Can you work these out from the model? Positions are in its coordinate system, mm. A direction names the side the tool comes from. Round coordinates to 2 decimals unless told otherwise and drop trailing zeros. Loops run counter-clockwise (first coordinate to the right, second up) from the corner with the lowest first, then second, coordinate; pieces in that order, holes last. Notation, with made-up numbers: (34.5, 2) -> (60.5, 2) arc R20 cw to (60.5, 14) -> close; hole circle Ø5 at (-29.5, 74). An arc over 180 degrees is marked (long way). Answer as a JSON object with one key per item and string values.
```python
from build123d import *

# Parameters (mm, degrees)
SKETCH_1_W          = 40
SKETCH_1_H          = 24
SKETCH_1_R          = 2
EXTRUDE_1_DEPTH     = 3
SKETCH_2_W          = 20
SKETCH_2_H          = 6
EXTRUDE_2_DEPTH     = 25
SKETCH_3_R          = 7.9375
CUT_EXTRUDE_1_DEPTH = 10


with BuildPart() as part:
    # 草图1 → 凸台-拉伸1 (new body)
    with BuildSketch(Plane(origin=(0, 0, 0), x_dir=(1, 0, 0), z_dir=(0, 1, 0))):
        Rectangle(SKETCH_1_W, SKETCH_1_H)
        with Locations((-14.8, -7.5)):
            Circle(SKETCH_1_R, mode=Mode.SUBTRACT)
        with Locations((14.8, -7.5)):
            Circle(SKETCH_1_R, mode=Mode.SUBTRACT)
        with Locations((-14.8, 7.5)):
            Circle(SKETCH_1_R, mode=Mode.SUBTRACT)
        with Locations((14.8, 7.5)):
            Circle(SKETCH_1_R, mode=Mode.SUBTRACT)
    extrude(amount=EXTRUDE_1_DEPTH)

    # 草图2 → 凸台-拉伸2 (add)
    with BuildSketch(Plane(origin=(0, 3, 0), x_dir=(1, 0, 0), z_dir=(0, 1, 0))):
        Rectangle(SKETCH_2_W, SKETCH_2_H)
    extrude(amount=EXTRUDE_2_DEPTH)

    # 草图3 → 切除-拉伸1 (cut)
    with BuildSketch(Plane.XY.offset(3)):
        with Locations((0, 17)):
            Circle(SKETCH_3_R)
    extrude(amount=-CUT_EXTRUDE_1_DEPTH, mode=Mode.SUBTRACT)


solid = part.part
```
Q1. We'd pull the mould along X, two halves only. Please class faces 6 (the flat face through (-10, 15, 0)), 7 (the cylindrical face through (4.27, 23.69, 0.04)), 8 (the flat face through (20, 1, 0)), 9 (the cylindrical face through (-13.725, 1.479, -9.186)): pulls with the +X half, pulls with the -X half, needs draft (parallel to the pull), parting line crosses it, or undercut.
Determined:
{"face 6": "pulls with the -X half", "face 7": "undercut", "face 8": "pulls with the +X half", "face 9": "undercut"}
Q2. If I drill on L1, parallel to Z at x = 14.8, y = 1.6; L2, parallel to X at y = 2.05, z = 7.5; L3, parallel to Y at x = 0, z = 1.05, over which ranges is the centre line in solid material (lowest first)? Write a range as [from, to].
Determined:
{"L1": "[-12, -9.5], [-5.5, 5.5], [9.5, 12]", "L2": "[-20, -16.8], [-12.8, 12.8], [16.8, 20]", "L3": "[0, 9.06], [24.94, 28]"}
Q3. I want a section at D-D, the plane z = -0.75. Write out the boundary of the cut face in (x, y) (1 decimal).
Determined:
{"outline": "(-20, 0) -> (20, 0) -> (20, 3) -> (10, 3) -> (10, 28) -> (-10, 28) -> (-10, 3) -> (-20, 3) -> close; hole circle Ø15.9 at (0, 17)"}
Q4. I'm going to push flat-ended pins straight in: pin 1 (8 mm diameter, centred on y = 24, z = 4, fed in from -X); pin 2 (16 mm diameter, centred on x = -2, y = 18.5, fed in from +Z); pin 3 (6.5 mm diameter, centred on y = 20.5, z = 1.5, fed in from +X). Where does each tip first touch, or does it pass through?
Determined:
{"pin 1": "x = -10", "pin 2": "z = 3", "pin 3": "x = 10"}
Q5. On a 3-axis mill with a long thin cutter (end or side, diameter ignored), from which of +Z, -Z, +X, -X, +Y, -Y can I reach the whole of each face in a straight line? I mean faces 1 (the cylindrical face through (12.802, 1.479, 7.412)), 2 (the flat face through (0, 1, -12)), 3 (the flat face through (10, 15, 0)), 4 (the flat face through (-5, 10, -3)), 5 (the flat face through (-5, 10, 3)). Say none if no direction works.
Determined:
{"face 1": "+Y, -Y", "face 2": "-Z, +X, -X, +Y, -Y", "face 3": "+Z, -Z, +X, +Y", "face 4": "-Z, +X, -X, +Y", "face 5": "+Z, +X, -X, +Y"}
Q6. I want a section at A-A, the plane x = 0. Write out the boundary of the cut face in (y, z), then the cut area to 3 significant figures.
Determined:
{"outline": "(0, -12) -> (3, -12) -> (3, -3) -> (9.06, -3) -> (9.06, 3) -> (3, 3) -> (3, 12) -> (0, 12) -> close; (24.94, -3) -> (28, -3) -> (28, 3) -> (24.94, 3) -> close", "area": "127 mm²"}
Q7. I want a section at B-B, the plane z = 7.5. Write out the boundary of the cut face in (x, y).
Determined:
{"outline": "(-20, 0) -> (-16.8, 0) -> (-16.8, 3) -> (-20, 3) -> close; (-12.8, 0) -> (12.8, 0) -> (12.8, 3) -> (-12.8, 3) -> close; (16.8, 0) -> (20, 0) -> (20, 3) -> (16.8, 3) -> close"}
Q8. I want a section at C-C, the plane y = 17. Write out the boundary of the cut face in (x, z), then the cut area to 4 significant figures.
Determined:
{"outline": "(-10, -3) -> (-7.94, -3) -> (-7.94, 3) -> (-10, 3) -> close; (7.94, -3) -> (10, -3) -> (10, 3) -> (7.94, 3) -> close", "area": "24.75 mm²"}
